Source: CAD feature listing. Evaluate the final solid. Frame: model axes, mm. Give positions to 0.01 mm unless a question says otherwise; leave off trailing zeros. Order: outer loops, then holes, each group sorted by start corner. A loop starts at its lowest first (then second) coordinate and runs counter-clockwise, first axis right, second up. Notation, with made-up numbers: M 28.25,45.5 L 65.25,45.5 A15 ccw 65.25,71.5 Z; hole C 78.5,23 d10. An arc over 180 degrees is marked long. Answer in a Markdown table with one row per item. Add a question column.
(1) Section query A-A, the plane y = 4.25. Return loops of the section in (x, z).
(2) Mould query, pull axis Z, two halves, no side actions, for faces 1 (the face through (12.522, 12.697, -25.121)), 2 (the face through (13, 13, 0)), 3 (the face through (13, 13, -50.8)), 4 (the face through (0, 16, -25)). Classes: pulls with the +Z half, pulls with the -Z half, needs draft (parallel to the pull), parting line crosses it, or undercut.
(3) Section query D-D, the plane y = 7. Return loops of the section in (x, z), plus the area to 3 significant figures.
(4) Section query B-B, the plane x = 20. Return loops of the section in (y, z).
(5) Material intervals for line 1 along Z through (x, y) = (6.5, 7.25); line 2 along Z through (x, y) = (14.5, 3); line 3 along Y through (x, z) = (12.25, -14.5), sorted ascending.
(6) Section query C-C, the plane z = -25.4. Return loops of the section in (x, y).
from build123d import *

# Parameters (mm, degrees)
BOSS_EXTRUDE1_DEPTH = 25.4


with BuildPart() as part:
    # Sketch1 → Boss-Extrude1 (new body)
    with BuildSketch(Plane(origin=(0, 0, 0), x_dir=(0, 0, -1), z_dir=(1, 0, 0))):
        with BuildLine():
            Line((0, 25.4), (0, 0))
            Line((0, 0), (2.459031877, 0))
            Line((2.459031877, 0), (12.7, 0))
            ThreePointArc((12.7, 0), (25.4, 12.7), (38.1, 0))
            Line((38.1, 0), (50.8, 0))
            Line((50.8, 0), (50.8, 25.4))
            Line((50.8, 25.4), (0, 25.4))
        make_face()
    extrude(amount=BOSS_EXTRUDE1_DEPTH)


solid = part.part
Values follow:
| question | item | result |
|---|---|---|
| 1 | outline | M 0,-50.8 L 25.4,-50.8 L 25.4,-37.37 L 0,-37.37 Z; M 0,-13.43 L 25.4,-13.43 L 25.4,0 L 0,0 Z |
| 2 | face 1 | undercut |
| 2 | face 2 | pulls with the +Z half |
| 2 | face 3 | pulls with the -Z half |
| 2 | face 4 | needs draft |
| 3 | outline | M 0,-50.8 L 25.4,-50.8 L 25.4,-36 L 0,-36 Z; M 0,-14.8 L 25.4,-14.8 L 25.4,0 L 0,0 Z |
| 3 | area | 752 mm² |
| 4 | outline | M 0,-50.8 L 25.4,-50.8 L 25.4,0 L 0,0 L 0,-12.7 A12.7 cw 0,-38.1 Z |
| 5 | line 1 | z = -50.8 to -35.83, -14.97 to 0 |
| 5 | line 2 | z = -50.8 to -37.74, -13.06 to 0 |
| 5 | line 3 | y = 6.52 to 25.4 |
| 6 | outline | M 0,12.7 L 25.4,12.7 L 25.4,25.4 L 0,25.4 Z |
